```python
from build123d import *

# Parameters (mm, degrees)
SKETCH1_R            = 9
BOSS_EXTRUDE1_DEPTH  = 4
M4_CLEARANCE_HOLE1_D = 4.3


with BuildPart() as part:
    # Sketch1 → Boss-Extrude1 (new body)
    with BuildSketch(Plane.XY):
        with BuildLine():
            ThreePointArc((-70, 145), (-35, 110), (0, 145))
            ThreePointArc((0, 145), (-35, 180), (-70, 145))
        make_face()
        with Locations((-35, 145)):
            Circle(SKETCH1_R, mode=Mode.SUBTRACT)
    extrude(amount=BOSS_EXTRUDE1_DEPTH)

    # M4 Clearance Hole1 (through all)
    with Locations(Plane.XY.offset(4)):
        with Locations((-35, 170), (-10, 145), (-35, 120), (-60, 145)):
            Hole(M4_CLEARANCE_HOLE1_D / 2)


solid = part.part
```
Work out the finished part from the listing and answer in its coordinate system (mm). Give positions to 0.01 mm unless a question says otherwise; leave off trailing zeros. Write each loop counter-clockwise with the first axis right and the second up, starting at its lowest first coordinate (ties: lowest second). Pieces come first, ordered by that corner, then holes.
(1) The mould has two halves that part along X. Classify faces 1 (the flat face through (-28, 138, 4)), 2 (the cylindrical face through (-35.99, 118.09, 1.97)), 3 (the cylindrical face through (-59.53, 142.9, 1.97)), 4 (the cylindrical face through (-42.587, 110.832, 1.972)): pulls with the +X half, pulls with the -X half, needs draft (parallel to the pull), parting line crosses it, or undercut.
Final values:
face 1: needs draft
face 2: undercut
face 3: undercut
face 4: parting line crosses it
(2) The part is cut by section D-D on x = -60. Write down the section's boundary in (y, z).
Final values:
outline: (120.51, 0) - (142.85, 0) - (142.85, 4) - (120.51, 4) - close; (147.15, 0) - (169.49, 0) - (169.49, 4) - (147.15, 4) - close
(3) Flat-ended cylindrical pins translate along their axes: pin 1 Ø1 at (x, z) = (-44, 0.5) entering from -Y; pin 2 Ø1 at (y, z) = (130.5, 2.5) entering from -X. Find the tip coordinate at first contact, or state that the pin passes through.
Final values:
pin 1: stops at y = 111.05
pin 2: stops at x = -67.08
(4) The part is cut by section B-B on y = 120. Write down the section's boundary in (x, z).
Final values:
outline: (-59.49, 0) - (-37.15, 0) - (-37.15, 4) - (-59.49, 4) - close; (-32.85, 0) - (-10.51, 0) - (-10.51, 4) - (-32.85, 4) - close
(5) The part is cut by section A-A on x = -35. Write down the section's boundary in (y, z), plus the area to 3 significant figures.
Final values:
outline: (110, 0) - (117.85, 0) - (117.85, 4) - (110, 4) - close; (122.15, 0) - (136, 0) - (136, 4) - (122.15, 4) - close; (154, 0) - (167.85, 0) - (167.85, 4) - (154, 4) - close; (172.15, 0) - (180, 0) - (180, 4) - (172.15, 4) - close
area: 174 mm2
(6) Straight lines are drawn through the part: line 1 (Y direction, x = -35, z = 2.8); line 2 (Y direction, x = -59, z = 1); line 3 (X direction, y = 170, z = 2.3). For each, find the intervals that lie inside material, in ascending order.
Final values:
line 1: y = 110 to 117.85, 122.15 to 136, 154 to 167.85, 172.15 to 180
line 2: y = 119.52 to 143.1, 146.9 to 170.48
line 3: x = -59.49 to -37.15, -32.85 to -10.51
(7) The part is cut by section C-C on z = 1.05. Write down the section's boundary in (x, y), plus the area to 3 significant figures.
Final values:
outline: circle Ø70 at (-35, 145); hole circle Ø4.3 at (-60, 145); hole circle Ø18 at (-35, 145); hole circle Ø4.3 at (-35, 120); hole circle Ø4.3 at (-35, 170); hole circle Ø4.3 at (-10, 145)
area: 3,540 mm2
